Here's how the part is built. I have some questions about the finished solid (model axes, mm). Coordinates: 2 decimals unless noted, no trailing zeros. Order: outer loops, then holes, each group sorted by start corner. A loop starts at its lowest first (then second) coordinate and runs counter-clockwise, first axis right, second up.
```python
from build123d import *

# Parameters (mm, degrees)
F1_DEPTH  = 30
F3_DEPTH  = 25
F5_R      = 1.5
F6_DEPTH  = 13.5
F8_DEPTH  = 30
F11_DEPTH = 15


with BuildPart() as f1:
    # F0 (on Top) → F1 (new body)
    with BuildSketch(Plane.XY):
        with BuildLine():
            Line((0, 0), (12.9903810568, -7.5))
            ThreePointArc((12.9903810568, -7.5), (12.9903810568, 7.5), (0, 15))
            Line((0, 15), (0, 0))
        make_face()
    extrude(amount=-F1_DEPTH)

    # F2 (on face) → F3 (cut)
    with BuildSketch(Plane(origin=(0, 0, -30), x_dir=(1, 0, 0), z_dir=(0, 0, -1))):
        with BuildLine():
            Line((0, 0), (9.9592921435, 5.75))
            ThreePointArc((9.9592921435, 5.75), (-9.9592921435, 5.75), (0, -11.5))
            Line((0, -11.5), (0, 0))
        make_face()
        with BuildLine():
            ThreePointArc((0, -11.5), (8.1317279836, -8.1317279836), (11.5, 0))
            ThreePointArc((11.5, 0), (11.1081470023, 2.9764190187), (9.9592921435, 5.75))
            Line((9.9592921435, 5.75), (0, 0))
            Line((0, 0), (0, -11.5))
        make_face()
    extrude(amount=-F3_DEPTH, mode=Mode.SUBTRACT)

    # F5 (on face) → F6 (cut, symmetric)
    with BuildSketch(Plane(origin=(0, 0, 0), x_dir=(0.8660254038, 0.5, 0), z_dir=(0.5, -0.8660254038, 0))):
        with Locations((11, -2.5)):
            Circle(F5_R)
    extrude(amount=F6_DEPTH, both=True, mode=Mode.SUBTRACT)

    # F7 (on face) → F8 (cut)
    with BuildSketch(Plane.XY):
        with BuildLine():
            ThreePointArc((0, 15), (0.2500347391, 14.9979159429), (0.5, 14.9916643506))
            Line((0.5, 14.9916643506), (0.5, 16.4106432348))
            Line((0.5, 16.4106432348), (-0.9136777371, 16.4106432348))
            Line((-0.9136777371, 16.4106432348), (-0.9136777371, -10.8329579234))
            Line((-0.9136777371, -10.8329579234), (14.0083907078, -10.8329579234))
            Line((14.0083907078, -10.8329579234), (14.0083907078, -7.5103978769))
            Line((14.0083907078, -7.5103978769), (13.2331621726, -7.0628194734))
            ThreePointArc((13.2331621726, -7.0628194734), (13.1135935799, -7.2824215355), (12.9903810568, -7.5))
            Line((12.9903810568, -7.5), (0, 0))
            Line((0, 0), (0, 15))
        make_face()
        with BuildLine():
            Line((13.2331621726, -7.0628194734), (0.5, 0.2886751346))
            Line((0.5, 0.2886751346), (0.5, 14.9916643506))
            ThreePointArc((0.5, 14.9916643506), (0.2500347391, 14.9979159429), (0, 15))
            Line((0, 15), (0, 0))
            Line((0, 0), (12.9903810568, -7.5))
            ThreePointArc((12.9903810568, -7.5), (13.1135935799, -7.2824215355), (13.2331621726, -7.0628194734))
        make_face()
    extrude(amount=-F8_DEPTH, mode=Mode.SUBTRACT)

    # F10 (on offset) → F11 (cut)
    with BuildSketch(Plane(origin=(0, 0, -29), x_dir=(1, 0, 0), z_dir=(0, 0, -1))):
        with BuildLine():
            ThreePointArc((9.2050485345, 3.9073112849), (8.6602540378, -5), (1.2186934341, -9.9254615164))
            Line((1.2186934341, -9.9254615164), (1.4928994567, -12.1586903576))
            ThreePointArc((1.4928994567, -12.1586903576), (10.6088111964, -6.125), (11.2761844548, 4.786456324))
            Line((11.2761844548, 4.786456324), (9.2050485345, 3.9073112849))
        make_face()
    extrude(amount=-F11_DEPTH, mode=Mode.SUBTRACT)


solid = f1.part
```
Q1. Will these pins go through, and if not, where does the flat tip stop? pin 1 (2 mm diameter, centred on y = -4.5, z = -9.5, fed in from -X); pin 2 (6 mm diameter, centred on x = 2.5, z = -10, fed in from -Y); pin 3 (3.5 mm diameter, centred on x = 7, y = 6, fed in from -Z).
Q2. If we section it at A-A on z = -23: Write out the boundary of the cut face in (x, y).
Q3. I need wall thicknesses on L1, parallel to Z at x = 2, y = 3.5; L2, parallel to Y at x = 10.25, z = -2; L3, parallel to X at y = 0.5, z = -11.5. Which ranges of each line are inside material? Lowest first, please.
Q4. We'd pull the mould along X, two halves only. Please class faces 1 (the flat face through (0.5, 12, -8)), 2 (the flat face through (6, 3, -5)), 3 (the cylindrical face through (8.31, 4.61, -2.43)): pulls with the +X half, pulls with the -X half, needs draft (parallel to the pull), parting line crosses it, or undercut.
Q5. If we section it at B-B on z = -3: Write out the boundary of the cut face in (x, y).
Q6. If we section it at C-C on z = -13: Write out the boundary of the cut face in (x, y), then the cut area to 3 significant figures.
Reply:
1. pin 1: stops at x = 10.2
1. pin 2: stops at y = 10.1
1. pin 3: stops at z = -5
2. outline: (0.5, 11.49) arc R11.5 cw to (1.4, 11.41) - (1.49, 12.16) arc R12.25 cw to (11.28, -4.79) - (10.59, -4.49) arc R11.5 cw to (10.2, -5.31) - (13.23, -7.06) arc R15 ccw to (0.5, 14.99) - close
3. L1: z = -5 to 0
3. L2: y = -5.34 to 1.42, 7.07 to 10.95
3. L3: x = 11.49 to 14.99
4. face 1: pulls with the -X half
4. face 2: needs draft
4. face 3: undercut
5. outline: (0.5, 0.29) - (13.23, -7.06) arc R15 ccw to (14.07, -5.2) - (2.53, 14.78) arc R15 ccw to (0.5, 14.99) - close; (6.54, 13.5) - (14.96, -1.08) arc R15 ccw to start
6. outline: (0.5, 11.49) arc R11.5 cw to (10.2, -5.31) - (13.23, -7.06) arc R15 ccw to (0.5, 14.99) - close
6. area: 93.6 mm2
